Geometry: final body of the model. Coordinates: model frame, mm. Give positions to 0.01 mm unless a question says otherwise; leave off trailing zeros. Loops run counter-clockwise (first coordinate to the right, second up) from the corner with the lowest first, then second, coordinate; pieces in that order, holes last.
1. First-contact query: P1, Ø8, axis at x = 16.5, z = -182.5, coming from the +Y side. Flat tip, straight axial feed; report the tip coordinate or a pass-through.
2. Section A-A, the plane y = 83. Output: boundary loops of the cut face in (x, z).
3. Material intervals for line 1 along Z through (x, y) = (11, 123); line 2 along Y through (x, z) = (14.25, 354.5); line 3 along X through (y, z) = (-59, -101), sorted ascending.
from build123d import *

# Parameters (mm, degrees)
F0_W     = 10
F0_H     = 350
F0_H_2   = 20
F0_H_3   = 190
F0_H_4   = 200
F0_W_2   = 390
F1_DEPTH = 10
F2_DEPTH = 20


with BuildPart() as f1:
    # F0 (on Right) → F1 (new body)
    with BuildSketch(Plane.YZ):
        with Locations((190.124774985, 511.8865245837)):
            Rectangle(F0_W, F0_H)
        with Locations((190.124774985, 326.8865245837)):
            Rectangle(F0_W, F0_H_2)
        with Locations((190.124774985, 221.8865245837)):
            Rectangle(F0_W, F0_H_3)
        with Locations((190.124774985, 116.8865245837)):
            Rectangle(F0_W, F0_H_2)
        with Locations((190.124774985, 6.8865245837)):
            Rectangle(F0_W, F0_H_4)
        with Locations((190.124774985, -103.1134754163)):
            Rectangle(F0_W, F0_H_2)
        with Locations((190.124774985, -213.1134754163)):
            Rectangle(F0_W, F0_H_4)
        with Locations((-9.875225015, -103.1134754163)):
            Rectangle(F0_W_2, F0_H_2)
        with Locations((-9.875225015, 116.8865245837)):
            Rectangle(F0_W_2, F0_H_2)
        with Locations((-9.875225015, 326.8865245837)):
            Rectangle(F0_W_2, F0_H_2)
    extrude(amount=F1_DEPTH)

    # F0 (on Right) → F2 (join)
    with BuildSketch(Plane.YZ):
        with Locations((-9.875225015, 511.8865245837)):
            Rectangle(F0_W_2, F0_H)
        with Locations((-9.875225015, 221.8865245837)):
            Rectangle(F0_W_2, F0_H_3)
        with Locations((-9.875225015, 6.8865245837)):
            Rectangle(F0_W_2, F0_H_4)
        with Locations((-9.875225015, -213.1134754163)):
            Rectangle(F0_W_2, F0_H_4)
    extrude(amount=F2_DEPTH)


solid = f1.part
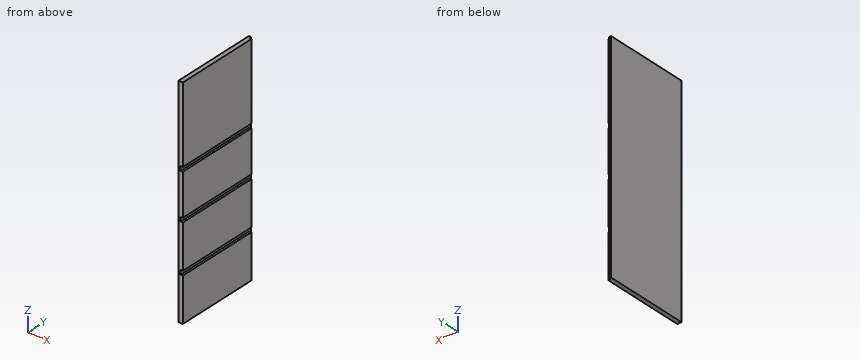
Answers below:
1. P1: stops at y = 185.12
2. outline: (0, -313.11) - (20, -313.11) - (20, -113.11) - (10, -113.11) - (10, -93.11) - (20, -93.11) - (20, 106.89) - (10, 106.89) - (10, 126.89) - (20, 126.89) - (20, 316.89) - (10, 316.89) - (10, 336.89) - (20, 336.89) - (20, 686.89) - (0, 686.89) - close
3. line 1: z = -313.11 to -113.11, -93.11 to 106.89, 126.89 to 316.89, 336.89 to 686.89
3. line 2: y = -204.88 to 185.12
3. line 3: x = 0 to 10
